from build123d import *

# Parameters (mm, degrees)
SKETCH_1_R          = 19
EXTRUDE_1_DEPTH     = 10
SKETCH_2_R          = 12.5
EXTRUDE_2_DEPTH     = 1
SKETCH_3_R          = 8.5
EXTRUDE_3_DEPTH     = 12.5
SKETCH_4_R          = 3.05
CUT_EXTRUDE_4_DEPTH = 2
SKETCH_7_R          = 5.25
CUT_EXTRUDE_3_DEPTH = 0.5
CUT_EXTRUDE_3_DRAFT = -45
FILLET_3_R          = 0.8
CHAMFER_1_SIZE      = 0.5
CHAMFER_2_SIZE      = 0.2


with BuildPart() as part:
    # Эскиз1 → Бобышка-Вытянуть1 (new body)
    with BuildSketch(Plane(origin=(0, 0, 0), x_dir=(1, 0, 0), z_dir=(0, 1, 0))):
        with Locations(Location((0, 0, 0), (0, 0, 270))):
            Circle(SKETCH_1_R)
    extrude(amount=EXTRUDE_1_DEPTH)

    # Эскиз2 → Бобышка-Вытянуть2 (add)
    with BuildSketch(Plane(origin=(0, 10, 0), x_dir=(1, 0, 0), z_dir=(0, 1, 0))):
        with Locations(Location((0, 0, 0), (0, 0, 270))):
            Circle(SKETCH_2_R)
    extrude(amount=EXTRUDE_2_DEPTH)

    # Эскиз3 → Бобышка-Вытянуть3 (add)
    with BuildSketch(Plane(origin=(0, 11, 0), x_dir=(1, 0, 0), z_dir=(0, 1, 0))):
        with Locations(Location((0, 0, 0), (0, 0, 270))):
            Circle(SKETCH_3_R)
    extrude(amount=EXTRUDE_3_DEPTH)

    # Эскиз4 → Вырез-Вытянуть4 (cut)
    with BuildSketch(Plane(origin=(0, 23.5, 0), x_dir=(1, 0, 0), z_dir=(0, 1, 0))):
        with Locations(Location((0, 0, 0), (0, 0, 270))):
            Circle(SKETCH_4_R)
    extrude(amount=-CUT_EXTRUDE_4_DEPTH, mode=Mode.SUBTRACT)


with BuildPart() as cut_extrude_3_tool:
    # Эскиз7 → Вырез-Вытянуть3 (with draft: the straight prism first)
    with BuildSketch(Plane.XZ):
        with Locations((0, 11.5)):
            Circle(SKETCH_7_R)
    extrude(amount=-CUT_EXTRUDE_3_DEPTH)
    # Вырез-Вытянуть3: the draft: its side faces are tilted about the plane it starts from
    cut_extrude_3_sides = [cut_extrude_3_tool.faces().sort_by_distance(p)[0] for p in [
        (-5.25, 0.25, 11.5),
    ]]
    draft(cut_extrude_3_sides, Plane.XZ, CUT_EXTRUDE_3_DRAFT)


with BuildPart() as part_1:
    add(part.part)

    # Вырез-Вытянуть3: cut by cut_extrude_3_tool
    add(cut_extrude_3_tool.part, mode=Mode.SUBTRACT)

    # Скругление3
    fillet_3_edges = [part_1.edges().sort_by_distance(p)[0] for p in [
        (-4.75, 0.5, 11.5),
        (-5.25, 0, 11.5),
    ]]
    fillet(fillet_3_edges, radius=FILLET_3_R)

    # Фаска1
    chamfer_1_edges = [part_1.edges().sort_by_distance(p)[0] for p in [
        (0, 23.5, -8.5),
    ]]
    chamfer(chamfer_1_edges, length=CHAMFER_1_SIZE)

    # Фаска2
    chamfer_2_edges = [part_1.edges().sort_by_distance(p)[0] for p in [
        (0, 23.5, -3.05),
    ]]
    chamfer(chamfer_2_edges, length=CHAMFER_2_SIZE)


solid = part_1.part
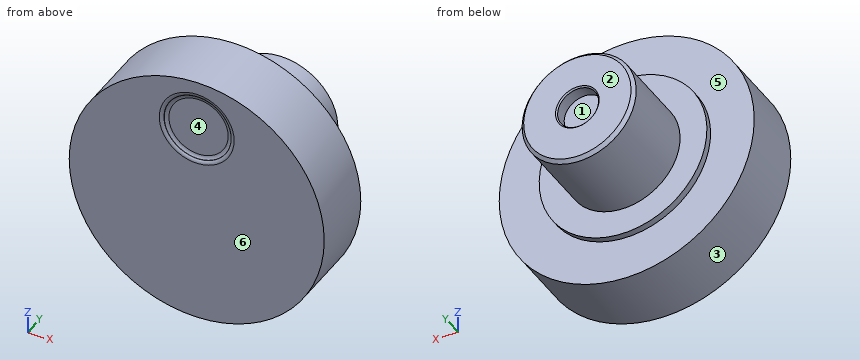
Here's how the part is built. I have some questions about the finished solid (model axes, mm). Face numbers are marked on the shaded views. A direction names the side the tool comes from. Give positions to 0.01 mm unless a question says otherwise; leave off trailing zeros. Order: outer loops, then holes, each group sorted by start corner. A loop starts at its lowest first (then second) coordinate and runs counter-clockwise, first axis right, second up. Notation, with made-up numbers: (75.25, -38) -> (131.25, -38) arc R22 cw to (131.25, -17) -> close; hole circle Ø10 at (-14.75, 81). An arc over 180 degrees is marked (long way). Use a Markdown table: item, result. Add a question column.
Item 1: I need wall thicknesses on line 1 (X direction, y = 22.3, z = 0); line 2 (Y direction, x = -7, z = 12.5); line 3 (Y direction, x = -7.5, z = -6). Which ranges of each line are inside material? Lowest first, please.
Item 2: If we mould it in two halves opening along Z, with no side actions, what happens to the marked faces 1, 2, 3 and 4? For each: pulls with the +Z half, pulls with the -Z half, needs draft (parallel to the pull), parting line crosses it, or undercut.
Item 3: Imagine slicing it at A-A on z = 0. Please give me the cut outline in (x, y).
Item 4: Imagine slicing it at B-B on x = 0. Please give me the cut outline in (y, z), plus the area to 3 significant figures.
Item 5: For the marked faces 5 and 6, which set-ups out of +Z, -Z, +X, -X, +Y, -Y let a thin tool reach every point of the face, with its end or its side?
Item 6: Will these pins go through, and if not, where does the flat tip stop? pin 1 (5 mm diameter, centred on x = 0, z = 0, fed in from +Y); pin 2 (8 mm diameter, centred on x = 4, y = 18, fed in from +Z); pin 3 (1.5 mm diameter, centred on y = 9.5, z = 8.5, fed in from +X); pin 4 (1 mm diameter, centred on y = 12, z = -13, fed in from +X).
Item 7: Imagine slicing it at D-D on z = 11.5. Please give me the cut outline in (x, y).
Item 8: Imagine slicing it at C-C on y = 4. Please give me the cut outline in (x, z).
Data:
| question | item | result |
|---|---|---|
| 1 | line 1 | x = -8.5 to -3.05, 3.05 to 8.5 |
| 1 | line 2 | y = 0 to 10 |
| 1 | line 3 | y = 0 to 11 |
| 2 | face 1 | undercut |
| 2 | face 2 | needs draft |
| 2 | face 3 | parting line crosses it |
| 2 | face 4 | undercut |
| 3 | outline | (-19, 0) -> (19, 0) -> (19, 10) -> (12.5, 10) -> (12.5, 11) -> (8.5, 11) -> (8.5, 23) -> (8, 23.5) -> (3.25, 23.5) -> (3.05, 23.3) -> (3.05, 21.5) -> (-3.05, 21.5) -> (-3.05, 23.3) -> (-3.25, 23.5) -> (-8, 23.5) -> (-8.5, 23) -> (-8.5, 11) -> (-12.5, 11) -> (-12.5, 10) -> (-19, 10) -> close |
| 4 | outline | (0, -19) -> (10, -19) -> (10, -12.5) -> (11, -12.5) -> (11, -8.5) -> (23, -8.5) -> (23.5, -8) -> (23.5, -3.25) -> (23.3, -3.05) -> (21.5, -3.05) -> (21.5, 3.05) -> (23.3, 3.05) -> (23.5, 3.25) -> (23.5, 8) -> (23, 8.5) -> (11, 8.5) -> (11, 12.5) -> (10, 12.5) -> (10, 19) -> (0, 19) -> (0, 17.08) arc R0.8 ccw to (0.23, 16.52) -> (0.27, 16.48) arc R0.8 cw to (0.5, 15.92) -> (0.5, 7.08) arc R0.8 cw to (0.27, 6.52) -> (0.23, 6.48) arc R0.8 ccw to (0, 5.92) -> close |
| 4 | area | 600 mm² |
| 5 | face 5 | +Y |
| 5 | face 6 | +Z, -Z, +X, -X, -Y |
| 6 | pin 1 | stops at y = 21.5 |
| 6 | pin 2 | stops at z = 8.5 |
| 6 | pin 3 | stops at x = 17.35 |
| 6 | pin 4 | passes through |
| 7 | outline | (-15.12, 0) -> (-5.58, 0) arc R0.8 ccw to (-5.02, 0.23) -> (-4.98, 0.27) arc R0.8 cw to (-4.42, 0.5) -> (4.42, 0.5) arc R0.8 cw to (4.98, 0.27) -> (5.02, 0.23) arc R0.8 ccw to (5.58, 0) -> (15.12, 0) -> (15.12, 10) -> (4.9, 10) -> (4.9, 11) -> (-4.9, 11) -> (-4.9, 10) -> (-15.12, 10) -> close |
| 8 | outline | circle Ø38 at (0, 0) |
